```python
from build123d import *

# Parameters (mm, degrees)
BOSS_EXTRUDE1_DEPTH = 19
SKETCH2_R           = 11
CUT_EXTRUDE1_DEPTH  = 19
SKETCH3_W           = 64
SKETCH3_H           = 64
BOSS_EXTRUDE2_DEPTH = 45
SKETCH10_W          = 38
SKETCH10_H          = 51
CUT_EXTRUDE2_DEPTH  = 51
BOSS_EXTRUDE3_DEPTH = 38


with BuildPart() as part:
    # Sketch1 → Boss-Extrude1 (new body)
    with BuildSketch(Plane(origin=(0, 0, 0), x_dir=(1, 0, 0), z_dir=(0, 1, 0))):
        with BuildLine():
            Line((0, 32), (114, 32))
            ThreePointArc((114, 32), (146, 0), (114, -32))
            Line((114, -32), (0, -32))
            ThreePointArc((0, -32), (-32, 0), (0, 32))
        make_face()
    extrude(amount=BOSS_EXTRUDE1_DEPTH)

    # Sketch2 → Cut-Extrude1 (cut)
    with BuildSketch(Plane(origin=(0, 19, 0), x_dir=(1, 0, 0), z_dir=(0, 1, 0))):
        Circle(SKETCH2_R)
        with Locations((114, 0)):
            Circle(SKETCH2_R)
    extrude(amount=-CUT_EXTRUDE1_DEPTH, mode=Mode.SUBTRACT)

    # Sketch3 → Boss-Extrude2 (add)
    with BuildSketch(Plane(origin=(0, 19, 0), x_dir=(1, 0, 0), z_dir=(0, 1, 0))):
        with Locations((57, 0)):
            Rectangle(SKETCH3_W, SKETCH3_H)
    extrude(amount=BOSS_EXTRUDE2_DEPTH)

    # Sketch10 → Cut-Extrude2 (cut)
    with BuildSketch(Plane(origin=(0, 64, 0), x_dir=(1, 0, 0), z_dir=(0, 1, 0))):
        with Locations((57, -6.5)):
            Rectangle(SKETCH10_W, SKETCH10_H)
    extrude(amount=-CUT_EXTRUDE2_DEPTH, mode=Mode.SUBTRACT)

    # Sketch11 → Boss-Extrude3 (add)
    with BuildSketch(Plane.ZY.offset(-76)):
        Polygon((-19, 64), (32, 13), (-19, 13), align=None)
    extrude(amount=BOSS_EXTRUDE3_DEPTH)


solid = part.part
```
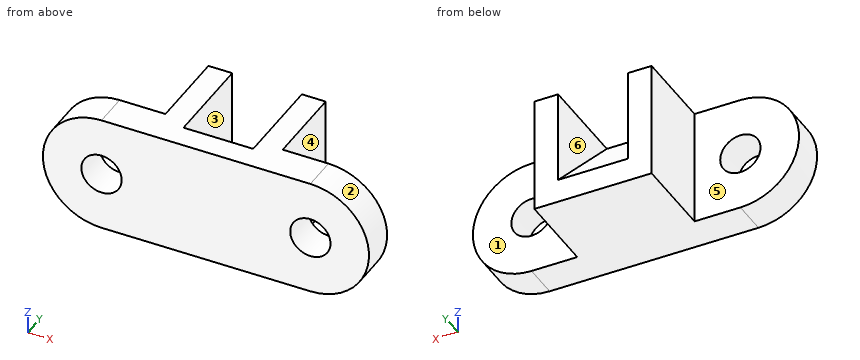
CAD build for the part. Positions are in the model's coordinates, mm. Face numbers are marked on the shaded views. A direction names the side the tool comes from. Coordinates: 2 decimals unless noted, no trailing zeros. Write each loop counter-clockwise with the first axis right and the second up, starting at its lowest first coordinate (ties: lowest second). Pieces come first, ordered by that corner, then holes.
(1) Cut at C-C, the plane y = 15. List the corners of the cut face in (x, z), and give its area (3 significant figures).
(2) Cut at D-D, the plane z = 18.5. List the corners of the cut face in (x, y), and give its area (3 significant figures).
(3) Cut at B-B, the plane y = 57. List the corners of the cut face in (x, z).
(4) Two-plate mould, pull along X, no slides. Class the marked faces 1, 2 and 3: +X half, -X half, draft (parallel to the pull), parting line (faces both ways), or undercut.
(5) 3-axis set-ups, long thin cutter, end or side, ignore diameter. For the marked faces 4, 5 and 6: which of +Z, -Z, +X, -X, +Y, -Y reach the whole face in a straight line?
(6) Drill centre lines: probe 1 along X at (y, z) = (12, 0); probe 2 along X at (y, z) = (60.5, 11); probe 3 along Z at (x, y) = (114, 6). Where is each one in solid material? Low to high.
(7) Cut at A-A, the plane z = 0. List the corners of the cut face in (x, y), and give its area (3 significant figures).
(8) Flat gauge pins, fed straight in: pin 1 (13 mm diameter, centred on x = 0, z = 0, fed in from +Y); pin 2 (3 mm diameter, centred on y = 52.5, z = 8, fed in from -X); pin 3 (6 mm diameter, centred on y = 10.5, z = 25, fed in from +X); pin 4 (8 mm diameter, centred on x = -7, y = 13, fed in from +Z). Where does each tip first touch, or does it go through?
Geometry says:
1. outline: (0, -32) - (114, -32) arc R32 ccw to (114, 32) - (76, 32) - (76, 30) - (38, 30) - (38, 32) - (0, 32) arc R32 ccw to start; hole circle Ø22 at (0, 0); hole circle Ø22 at (114, 0)
1. area: 9,680 mm2
2. outline: (-26.11, 0) - (140.11, 0) - (140.11, 19) - (89, 19) - (89, 64) - (76, 64) - (76, 26.5) - (38, 26.5) - (38, 64) - (25, 64) - (25, 19) - (-26.11, 19) - close
2. area: 4,610 mm2
3. outline: (25, -32) - (89, -32) - (89, 32) - (76, 32) - (76, -12) - (38, -12) - (38, 32) - (25, 32) - close
4. face 1: draft
4. face 2: +X half
4. face 3: undercut
5. face 4: +Z, -Z, +X, +Y
5. face 5: +Z, -Z, -X, +Y
5. face 6: +Z, +Y
6. probe 1: x = -32 to -11, 11 to 103, 125 to 146
6. probe 2: x = 25 to 38, 76 to 89
6. probe 3: z = -32 to -11, 11 to 32
7. outline: (-32, 0) - (-11, 0) - (-11, 19) - (-32, 19) - close; (11, 0) - (103, 0) - (103, 19) - (89, 19) - (89, 64) - (76, 64) - (76, 45) - (38, 45) - (38, 64) - (25, 64) - (25, 19) - (11, 19) - close; (125, 0) - (146, 0) - (146, 19) - (125, 19) - close
7. area: 4,700 mm2
8. pin 1: passes through
8. pin 2: stops at x = 25
8. pin 3: stops at x = 137.24
8. pin 4: stops at z = 31.86
